Read the model definition and answer for the solid it produces. Units are mm, in the model's axes. A direction names the side the tool comes from. Coordinates: 2 decimals unless noted, no trailing zeros. Order: outer loops, then holes, each group sorted by start corner. A loop starts at its lowest first (then second) coordinate and runs counter-clockwise, first axis right, second up. Notation, with made-up numbers: (20.25, 22.5) - (36.25, 22.5) arc R29 cw to (36.25, 58.5) - close; hole circle Ø10 at (73, 80.25). An arc over 180 degrees is marked (long way). Use one line per item in the form item = value.
```python
from build123d import *

# Parameters (mm, degrees)
CROQUIS1_R              = 1.5
SALIENTE_EXTRUIR1_DEPTH = 36
CORTAR_EXTRUIR1_DEPTH   = 6.3
MATRIZL1_COUNT          = 3
MATRIZL1_PITCH          = 12
CROQUIS3_R              = 2.25
CORTAR_EXTRUIR2_DEPTH   = 42.623310777
CHAFL_N1_SIZE           = 2.5
REDONDEO1_R             = 3
REDONDEO2_R             = 1


with BuildPart() as part:
    # Croquis1 → Saliente-Extruir1 (new body)
    with BuildSketch(Plane.XY):
        with BuildLine():
            Line((12.75, 7.897114317), (5.133974596, 3.5))
            Line((5.133974596, 3.5), (-10, 3.5))
            Line((-10, 3.5), (-10, -4))
            Line((-10, -4), (14.4, -4))
            Line((14.4, -4), (14.4, -0.5))
            Line((14.4, -0.5), (15, -0.5))
            ThreePointArc((15, -0.5), (19.346666218, 5.164685703), (12.75, 7.897114317))
        make_face()
        with Locations((15, 4)):
            Circle(CROQUIS1_R, mode=Mode.SUBTRACT)
    extrude(amount=-SALIENTE_EXTRUIR1_DEPTH)

    # Croquis2 → Cortar-Extruir1 (cut)
    with BuildSketch(Plane.XY):
        with BuildLine():
            Line((14.4, -0.842600764), (15, -0.5))
            ThreePointArc((15, -0.5), (19.346666218, 5.164685703), (12.75, 7.897114317))
            Line((12.75, 7.897114317), (5.133974596, 3.5))
            Line((5.133974596, 3.5), (11.80761005, 0.309549003))
            ThreePointArc((11.80761005, 0.309549003), (13.018228657, -0.459076642), (14.4, -0.842600764))
        make_face()
    cortar_extruir1 = extrude(amount=-CORTAR_EXTRUIR1_DEPTH, mode=Mode.SUBTRACT)

    # MatrizL1: Cortar-Extruir1 ×3
    with Locations(*[(0, 0, -i * MATRIZL1_PITCH) for i in range(1, MATRIZL1_COUNT)]):
        add(cortar_extruir1, mode=Mode.SUBTRACT)

    # Croquis3 → Cortar-Extruir2 (cut, through all)
    with BuildSketch(Plane(origin=(0, 3.5, 0), x_dir=(1, 0, 0), z_dir=(0, 1, 0))):
        with Locations(Location((-2, 28, 0), (0, 0, 270))):
            Circle(CROQUIS3_R)
        with Locations(Location((-2, 8, 0), (0, 0, 270))):
            Circle(CROQUIS3_R)
    extrude(amount=-CORTAR_EXTRUIR2_DEPTH, mode=Mode.SUBTRACT)

    # Chaflán1
    chafl_n1_edges = [part.edges().sort_by_distance(p)[0] for p in [
        (-2, 3.5, -30.25),
        (-2, 3.5, -10.25),
    ]]
    chamfer(chafl_n1_edges, length=CHAFL_N1_SIZE)

    # Redondeo1
    redondeo1_edges = [part.edges().sort_by_distance(p)[0] for p in [
        (-10, -0.25, -36),
        (-10, -0.25, 0),
    ]]
    fillet(redondeo1_edges, radius=REDONDEO1_R)

    # Redondeo2
    redondeo2_edges = [part.edges().sort_by_distance(p)[0] for p in [
        (-10, 3.5, -18),
        (-9.121320344, 3.5, -0.878679656),
        (-9.121320344, 3.5, -35.121320344),
        (-0.933012702, 3.5, -36),
        (-0.933012702, 3.5, 0),
    ]]
    fillet(redondeo2_edges, radius=REDONDEO2_R)


solid = part.part
```
(1) The mould has two halves that part along Z. Classify faces 1 (the flat face through (8.42, 1.93, -3.11)), 2 (the cylindrical face through (-0.848, 3.215, -35.699)), 3 (the cylindrical face through (13, -0.45, -15.11)): +Z half, -Z half, draft (parallel to the pull), parting line (faces both ways), or undercut.
Answer list:
face_1 = draft
face_2 = -Z half
face_3 = undercut
(2) Which of the six approach directions +Z, -Z, +X, -X, +Y, -Y give full straight-line access (tool end or side, diameter ignored) to faces 4 (the cylindrical face through (13, -0.45, -3.11)), 5 (the flat face through (14.4, -2, -18)), 6 (the flat face through (12, 4, -24)), 7 (the flat face through (6, 1, -36))?
Answer list:
face_4 = +Z, +X, +Y
face_5 = +Z, -Z, +X, -Y
face_6 = +X, +Y
face_7 = -Z, +X, -X, +Y, -Y
(3) Given pin 1 Ø6 at (x, y) = (11.5, 5.5) entering from +Z; pin 2 Ø3 at (y, z) = (-1.5, -24.5) entering from +X; pin 3 Ø2 at (x, z) = (16, -7.5) entering from -Y, each flat-ended and moving along its own axis, determine where each tip first touches the part or whether it passes through.
Answer list:
pin_1 = -6.3
pin_2 = 16.89
pin_3 = -0.5
(4) Straight lines are drawn through the part: L1, parallel to Z at x = 16.5, y = 5.75; L2, parallel to Y at x = 15, z = -9.15; L3, parallel to X at y = 3.75, z = -33.5. For each, find the intervals that lie inside material, in ascending order.
Answer list:
L1 = -36 to -30.3, -24 to -18.3, -12 to -6.3
L2 = -0.5 to 2.5, 5.5 to 8.5
L3 = 5.57 to 13.52, 16.48 to 19.49
(5) Section A-A, the plane z = -19.5 is taken. Write down the section's boundary in (x, y), then the cut area to 3 significant figures.
Answer list:
outline = (-10, -4) - (14.4, -4) - (14.4, -0.5) - (15, -0.5) arc R4.5 ccw (long way) to (12.75, 7.9) - (5.13, 3.5) - (-9, 3.5) arc R1 ccw to (-10, 2.5) - close; hole circle Ø3 at (15, 4)
area = 237 mm2
(6) Section D-D, the plane z = -28 is taken. Write down the section's boundary in (x, y).
Answer list:
outline = (-10, -4) - (-4.25, -4) - (-4.25, 1) - (-6.75, 3.5) - (-9, 3.5) arc R1 ccw to (-10, 2.5) - close; (0.25, -4) - (14.4, -4) - (14.4, -0.84) arc R4.88 cw to (11.81, 0.31) - (5.13, 3.5) - (2.75, 3.5) - (0.25, 1) - close
(7) Section B-B, the plane x = -2 is taken. Write down the section's boundary in (y, z).
Answer list:
outline = (-4, -36) - (2.5, -36) arc R1 ccw to (3.5, -35) - (3.5, -32.75) - (1, -30.25) - (-4, -30.25) - close; (-4, -25.75) - (1, -25.75) - (3.5, -23.25) - (3.5, -12.75) - (1, -10.25) - (-4, -10.25) - close; (-4, -5.75) - (1, -5.75) - (3.5, -3.25) - (3.5, -1) arc R1 ccw to (2.5, 0) - (-4, 0) - close
(8) Section C-C, the plane y = 4 is taken. Write down the section's boundary in (x, z), then the cut area to 3 significant figures.
Answer list:
outline = (6, -36) - (13.5, -36) - (13.5, -30.3) - (6, -30.3) - close; (6, -24) - (13.5, -24) - (13.5, -18.3) - (6, -18.3) - close; (6, -12) - (13.5, -12) - (13.5, -6.3) - (6, -6.3) - close; (16.5, -36) - (19.5, -36) - (19.5, -30.3) - (16.5, -30.3) - close; (16.5, -24) - (19.5, -24) - (19.5, -18.3) - (16.5, -18.3) - close; (16.5, -12) - (19.5, -12) - (19.5, -6.3) - (16.5, -6.3) - close
area = 180 mm2
